```python
from build123d import *

# Parameters (mm, degrees)
F0_R     = 8.964433
F1_DEPTH = 25.4
F2_DEPTH = 7.366
F4_DEPTH = 7.62


with BuildPart() as f1:
    # F0 (on Front) → F1 (new body)
    with BuildSketch(Plane.XZ):
        with BuildLine():
            ThreePointArc((-9.938305, -12.372125), (-2.792256, -7.934724), (0, 0))
            ThreePointArc((0, 0), (-3.165972, 8.378736), (-11.081682, 12.570171))
            ThreePointArc((-11.081682, 12.570171), (-25.326984, -0.580201), (-9.938305, -12.372125))
        make_face()
        with Locations((-12.670138, 0)):
            Circle(F0_R, mode=Mode.SUBTRACT)
    extrude(amount=F1_DEPTH)

    # F0 (on Front) → F2 (join)
    with BuildSketch(Plane.XZ):
        with BuildLine():
            ThreePointArc((-11.081682, 12.570171), (-3.165972, 8.378736), (0, 0))
            ThreePointArc((0, 0), (-2.792256, -7.934724), (-9.938305, -12.372125))
            Line((-9.938305, -12.372125), (20.246768, -12.57116))
            Line((20.246768, -12.57116), (19.755474, 12.570171))
            Line((19.755474, 12.570171), (-11.081682, 12.570171))
        make_face()
    extrude(amount=F2_DEPTH)

    # F3 (on face) → F4 (join)
    with BuildSketch(Plane.XZ.offset(7.366)):
        with BuildLine():
            Line((-0.452979, -3.357592), (20.001121, -0.000494))
            Line((20.001121, -0.000494), (0, 0))
            ThreePointArc((0, 0), (-0.113755, -1.694005), (-0.452979, -3.357592))
        make_face()
    extrude(amount=F4_DEPTH)


solid = f1.part
```
Geometry check sheet. Reference: the model listing, model coordinates, mm. A direction names the side the tool comes from. Give positions to 0.01 mm unless a question says otherwise; leave off trailing zeros. Write each loop counter-clockwise with the first axis right and the second up, starting at its lowest first coordinate (ties: lowest second). Pieces come first, ordered by that corner, then holes.
1) Gauge pin test, flat ends, axial feed: pin 1 (2 mm diameter, centred on y = -4, z = -7, fed in from +X); pin 2 (6.5 mm diameter, centred on x = 11, z = -7.5, fed in from -Y); pin 3 (2.5 mm diameter, centred on x = 12, z = -1.5, fed in from -Y); pin 4 (4 mm diameter, centred on x = -11.5, z = -6.5, fed in from +Y). Record the tip position at first contact, or that the pin passes through.
2) Access from +Z, -Z, +X, -X, +Y, -Y to the whole of each face (thin tool, end or side, straight path). Record for faces 1 (the flat face through (8, -7.366, -8)), 2 (the flat face through (8, -7.366, 6)), 3 (the flat face through (5, -4, 12.57)).
3) Section check D-D, the plane z = 6. Record the boundary of the cut face in (x, y).
4) Material ranges on L1, parallel to Y at x = 1, z = 5.25; L2, parallel to X at y = -24, z = -7.75; L3, parallel to X at y = -8, z = 7, recorded low to high.
5) Section check C-C, the plane x = -21. Record the boundary of the cut face in (y, z), and give its area (3 significant figures).
6) Section check B-B, the plane y = -21.75. Record the boundary of the cut face in (x, z).
7) Release check for a two-part mould opening along Z. For faces 4 (the flat face through (9.631, -11.123, -1.703)), 5 (the cylindrical face through (-4.12, -12.52, 2.69)), 6 (the flat face through (2, 0, 0)) record: pulls with the +Z half, pulls with the -Z half, needs draft (parallel to the pull), parting line crosses it, or undercut.
8) Section check A-A, the plane z = 1.5. Record the boundary of the cut face in (x, y).
Computed:
1. pin 1: stops at x = 20.16
1. pin 2: stops at y = -7.37
1. pin 3: stops at y = -14.99
1. pin 4: passes through
2. face 1: -Z, +X, -Y
2. face 2: +Z, +X, -Y
2. face 3: +Z, +X, +Y, -Y
3. outline: (-23.83, -25.4) - (-19.33, -25.4) - (-19.33, 0) - (-23.83, 0) - close; (-6.01, -25.4) - (-1.51, -25.4) - (-1.51, -7.37) - (19.88, -7.37) - (19.88, 0) - (-6.01, 0) - close
4. L1: y = -7.37 to 0
4. L2: x = -22.69 to -17.18, -8.16 to -2.65
4. L3: x = -23.23 to -18.27, -7.07 to -2.11
5. outline: (-25.4, -9.55) - (0, -9.55) - (0, -3.31) - (-25.4, -3.31) - close; (-25.4, 3.31) - (0, 3.31) - (0, 9.55) - (-25.4, 9.55) - close
5. area: 317 mm2
6. outline: circle Ø25.34 at (-12.67, 0); hole circle Ø17.93 at (-12.67, 0)
7. face 4: pulls with the -Z half
7. face 5: undercut
7. face 6: needs draft
8. outline: (-25.25, -25.4) - (-21.51, -25.4) - (-21.51, 0) - (-25.25, 0) - close; (-3.83, -25.4) - (-0.09, -25.4) - (-0.09, -7.37) - (19.97, -7.37) - (19.97, 0) - (-3.83, 0) - close
